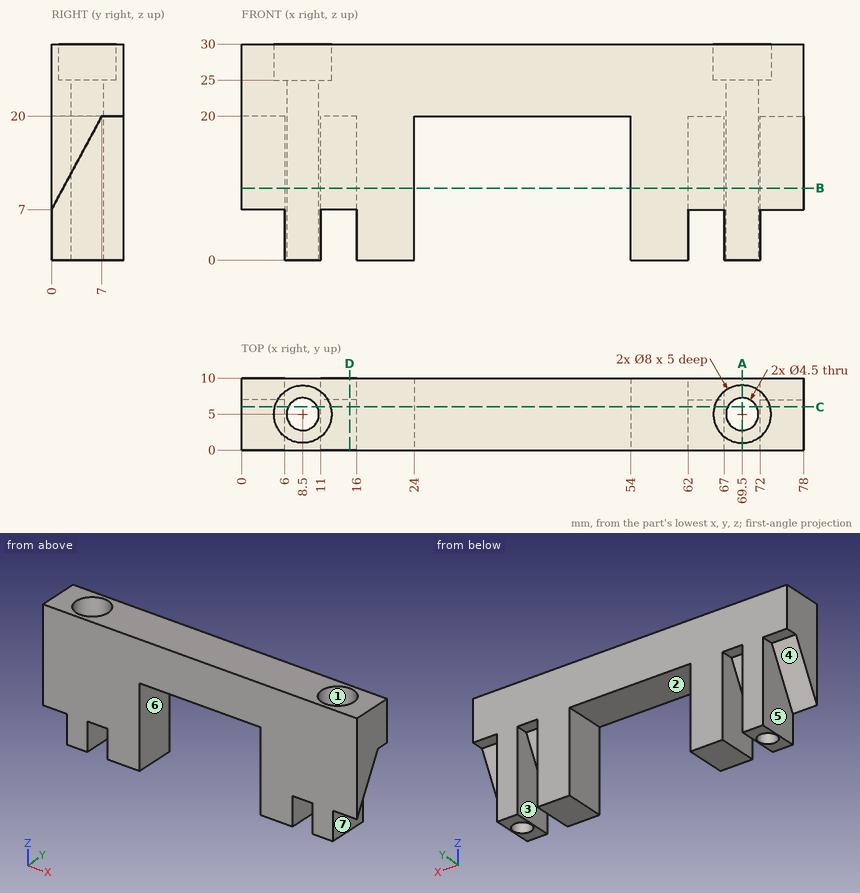
Check sheet for the drawn part. Datum: minimum x, y, z corner. Units: mm. A direction names the side the tool comes from. Coordinates: 2 decimals unless noted, no trailing zeros. Loops run counter-clockwise (first coordinate to the right, second up) from the corner with the lowest first, then second, coordinate; pieces in that order, holes last. Notation, with made-up numbers: (20, 68.5) -> (28, 68.5) arc R21 cw to (28, 79.5) -> close; hole circle Ø6 at (50, 37.5). An arc over 180 degrees is marked (long way). Answer in a Markdown table with one row per item.
1) Draft check along X on the marked faces 4, 5, 6 and 7. Enter one of: released by +X, released by -X, zero draft, split by the parting line, or undercut.
The answers:
| item | result |
|---|---|
| face 4 | zero draft |
| face 5 | released by -X |
| face 6 | undercut |
| face 7 | released by +X |
2) Section check B-B (z = 10). Record the cut outline in (x, y), and give its area (3 significant figures).
The answers:
| item | result |
|---|---|
| outline | (0, 0) -> (24, 0) -> (24, 10) -> (16, 10) -> (16, 1.62) -> (11, 1.62) -> (11, 10) -> (6, 10) -> (6, 1.62) -> (0, 1.62) -> close; (54, 0) -> (78, 0) -> (78, 1.62) -> (72, 1.62) -> (72, 10) -> (67, 10) -> (67, 1.62) -> (62, 1.62) -> (62, 10) -> (54, 10) -> close; hole circle Ø4.5 at (8.5, 5); hole circle Ø4.5 at (69.5, 5) |
| area | 264 mm2 |
3) Scan lines: line 1 along X through (y, z) = (2.25, 1.5); line 2 along X through (y, z) = (5.25, 28.5); line 3 along X through (y, z) = (5.25, 5). Record each from-to range of solid material in increasing order. Write a range as from..to.
The answers:
| item | result |
|---|---|
| line 1 | x = 6..11, 16..24, 54..62, 67..72 |
| line 2 | x = 0..4.51, 12.49..65.51, 73.49..78 |
| line 3 | x = 6..6.26, 10.74..11, 16..24, 54..62, 67..67.26, 71.74..72 |
4) Access from +Z, -Z, +X, -X, +Y, -Y to the whole of each face (thin tool, end or side, straight path). Record for the marked faces 1, 2 and 3.
The answers:
| item | result |
|---|---|
| face 1 | +Z |
| face 2 | -Z, +Y, -Y |
| face 3 | -Z, +Y |
5) Section check A-A (x = 69.5). Record the cut outline in (y, z).
The answers:
| item | result |
|---|---|
| outline | (0, 0) -> (2.75, 0) -> (2.75, 25) -> (1, 25) -> (1, 30) -> (0, 30) -> close; (7.25, 0) -> (10, 0) -> (10, 30) -> (9, 30) -> (9, 25) -> (7.25, 25) -> close |
6) Section check C-C (y = 6). Give the number of separate pieces and of enclosed holes in the cut face, and give its area (3 significant figures).
The answers:
| item | result |
|---|---|
| separate pieces | 3 |
| enclosed holes | 0 |
| area | 1,060 mm2 |
7) Depth check by flat-ended pin: P1, Ø2, axis at x = 30.5, y = 8, coming from the -Z side; P2, Ø3, axis at y = 6, z = 12.5, coming from the -X side; P3, Ø5, axis at y = 6.5, z = 9.5, coming from the +X side. Enter the tip coordinate at first touch or a pass-through.
The answers:
| item | result |
|---|---|
| P1 | stops at z = 20 |
| P2 | stops at x = 6 |
| P3 | stops at x = 72 |
8) Section check D-D (x = 15). Record the cut outline in (y, z).
The answers:
| item | result |
|---|---|
| outline | (0, 7) -> (7, 20) -> (10, 20) -> (10, 30) -> (0, 30) -> close |
